Autodesk Inventor part; units mm, degrees
ref_plane "YZ Plane" through (0, 0, 0) normal (1, 0, 0) x (0, 1, 0)
ref_plane "XZ Plane" through (0, 0, 0) normal (0, 1, 0) x (-1, 0, 0)
ref_plane "XY Plane" through (0, 0, 0) normal (0, 0, 1) x (1, 0, 0)
sketch "スケッチ1" plane through (0, 0, 0) normal (0, 0, 1) x (1, 0, 0)
  line L0 (-30, -32) -> (30, -32)
  line L1 (30, -32) -> (30, 32)
  line L2 (30, 32) -> (-30, 32)
  line L3 (-30, 32) -> (-30, -32)
  point P0 (0, 0)
  point P1 (0, -32)
  point P2 (-30, 0)
  dimension "d0" = 60
  dimension "d1" = 64
extrude "押し出し1" add sketch "スケッチ1" along normal blind 10
sketch "スケッチ2" plane through (0, 0, 10) normal (0, 0, 1) x (1, 0, 0)
  point P0 (0, 0)
  point P1 (-23, -12)
  dimension "d4" = 23
  dimension "d5" = 12
hole "穴1" at (-23, -12, 10) direction (0, 0, -1) diameter 5.5 end through all counterbore diameter 9.5 counterbore depth 5.5
pattern_linear "矩形状パターン1" count 2 spacing 24 along (0, 1, 0) count 2 spacing 46 along (1, 0, 0) of "穴1"
sketch "スケッチ3" plane through (0, 0, 10) normal (0, 0, 1) x (1, 0, 0)
  circle A0 centre (23, -12) radius 4.75
  circle A1 centre (-23, -12) radius 4.75
  point P0 (0, 0)
  point P1 (-23, 0)
  point P2 (23, 0)
hole "穴2" at (-23, 0, 10) at (23, 0, 10) direction (0, 0, -1) diameter 5 end through all
sketch "スケッチ4" plane through (0, 0, 10) normal (0, 0, 1) x (1, 0, 0)
  point P0 (0, 0)
  point P1 (0, 19.5)
  point P2 (0, -19.5)
  dimension "d26" = 19.5
  dimension "d27" = 19.5
hole "穴3" at (0, 19.5, 10) at (0, -19.5, 10) direction (0, 0, -1) diameter 3.242 end through all
sketch "スケッチ5" plane through (0, 0, 10) normal (0, 0, 1) x (1, 0, 0)
  circle A0 centre (0, -19.5) radius 1.621
  circle A1 centre (0, 19.5) radius 1.621
  point P0 (0, 0)
  point P1 (-19, 19.5)
  point P2 (-19, -19.5)
  dimension "d35" = 19
hole "穴4" at (-19, 19.5, 10) at (-19, -19.5, 10) direction (0, 0, -1) diameter 4 end through all
chamfer "面取り1" distance 2 angle 45 4 edges at (30, 32, 5) (30, -32, 5) (-30, -32, 5) (-30, 32, 5)
properties part number "03" material "A5052"
Geometry: final body of the model. Coordinates: model frame, mm. A direction names the side the tool comes from. Round coordinates to 2 decimals unless told otherwise and drop trailing zeros. Write each loop counter-clockwise with the first axis right and the second up, starting at its lowest first coordinate (ties: lowest second). Pieces come first, ordered by that corner, then holes.
Item 1: Set-up query: faces 1 (the face through (-27.71, 12.62, 7.21)), 2 (the face through (20.273, 12.358, 2.218)). Return all of +Z, -Z, +X, -X, +Y, -Y with unobstructed straight access to the full face (end or side cutting, diameter ignored); none if empty.
Item 2: Section query B-B (z = 3.75). Give the number of separate pieces and of enclosed holes in the cut face, plus the area to 3 significant figures.
Item 3: Section query C-C (x = 0). Return loops of the section in (y, z), plus the area to 3 significant figures.
Item 4: Pin query (flat end, axial travel): P1, Ø5, axis at x = -23, y = 12, coming from the -Z side; P2, Ø8, axis at x = 23, y = 0, coming from the +Z side; P3, Ø5, axis at x = 22.5, y = 11.5, coming from the +Z side. Return the tip coordinate at first contact, or that it passes through.
Item 5: Mould query, pull axis Y, two halves, no side actions, for faces 3 (the face through (29, -31, 5)), 4 (the face through (-30, 0, 5)), 5 (the face through (20.273, -11.642, 2.218)). Classes: +Y half, -Y half, draft (parallel to the pull), parting line (faces both ways), or undercut.
Item 6: Material intervals for L1, parallel to Y at x = 23, z = 8.7; L2, parallel to Y at x = 23, z = 1.4; L3, parallel to X at y = 12, z = 8.75, sorted ascending.
Item 7: Section query A-A (y = 0). Return loops of the section in (x, z), plus the area to 3 significant figures.
Item 8: Section query D-D (y = 12). Return loops of the section in (x, z), plus the area to 3 significant figures.
Completed:
1. face 1: +Z
1. face 2: +Z, -Z
2. separate pieces: 1
2. enclosed holes: 10
2. area: 3,660 mm2
3. outline: (-32, 0) - (-21.12, 0) - (-21.12, 10) - (-32, 10) - close; (-17.88, 0) - (17.88, 0) - (17.88, 10) - (-17.88, 10) - close; (21.12, 0) - (32, 0) - (32, 10) - (21.12, 10) - close
3. area: 575 mm2
4. P1: passes through
4. P2: stops at z = 10
4. P3: stops at z = 4.5
5. face 3: -Y half
5. face 4: draft
5. face 5: undercut
6. L1: y = -32 to -16.75, -7.25 to -2.5, 2.5 to 7.25, 16.75 to 32
6. L2: y = -32 to -14.75, -9.25 to -2.5, 2.5 to 9.25, 14.75 to 32
6. L3: x = -30 to -27.75, -18.25 to 18.25, 27.75 to 30
7. outline: (-30, 0) - (-25.5, 0) - (-25.5, 10) - (-30, 10) - close; (-20.5, 0) - (20.5, 0) - (20.5, 10) - (-20.5, 10) - close; (25.5, 0) - (30, 0) - (30, 10) - (25.5, 10) - close
7. area: 500 mm2
8. outline: (-30, 0) - (-25.75, 0) - (-25.75, 4.5) - (-27.75, 4.5) - (-27.75, 10) - (-30, 10) - close; (-20.25, 0) - (20.25, 0) - (20.25, 4.5) - (18.25, 4.5) - (18.25, 10) - (-18.25, 10) - (-18.25, 4.5) - (-20.25, 4.5) - close; (25.75, 0) - (30, 0) - (30, 10) - (27.75, 10) - (27.75, 4.5) - (25.75, 4.5) - close
8. area: 446 mm2
